```python
from build123d import *

# Parameters (mm, degrees)
SKETCH1_W                        = 69.85
SKETCH1_H                        = 19.05
MAIN_BODY_DEPTH                  = 3.175
CHIN_FEATURE_DEPTH               = 3.175
SKETCH10_W                       = 3.2258
SKETCH10_H                       = 6.35
CUT_FOR_TABS_DEPTH               = 4.175
CUT_FOR_LIP_MOTOR_APERTURE_DEPTH = 4.175
SKETCH12_R                       = 0.381
CUT_EXTRUDE1_DEPTH               = 4.175


with BuildPart() as part:
    # Sketch1 → main body (new body)
    with BuildSketch(Plane.XY):
        Rectangle(SKETCH1_W, SKETCH1_H)
    extrude(amount=MAIN_BODY_DEPTH)

    # Sketch9 → chin feature (add)
    with BuildSketch(Plane.XY.offset(3.175)):
        Polygon((-34.925, -9.525), (-34.925, -12.065), (-21.214947133, -17.145), (0, -17.145), (0, -9.525), align=None)
    chin_feature = extrude(amount=-CHIN_FEATURE_DEPTH)

    # mirror of chin feature: chin feature across plane
    add(chin_feature.mirror(Plane(origin=(0, 0, 0), x_dir=(0, 0, 1), z_dir=(1, 0, 0))))

    # Sketch10 → cut for tabs (cut, through all)
    with BuildSketch(Plane.XY.offset(3.175)):
        with Locations((-30.076100278, -4.050352196)):
            Rectangle(SKETCH10_W, SKETCH10_H)
        with Locations((19.20572281, -4.050352196)):
            Rectangle(SKETCH10_W, SKETCH10_H)
    extrude(amount=-CUT_FOR_TABS_DEPTH, mode=Mode.SUBTRACT)

    # Sketch11 → cut for lip motor aperture (cut, through all)
    with BuildSketch(Plane.XY.offset(3.175)):
        with BuildLine():
            Line((-23.576637278, 18.516146957), (-26.370637278, 18.516146957))
            Line((-26.370637278, 18.516146957), (-26.370637278, 14.520081328))
            ThreePointArc((-26.370637278, 14.520081328), (-23.470211189, 1.422172556), (-20.782637278, 14.565407781))
            Line((-20.782637278, 14.565407781), (-20.782637278, 18.516146957))
            Line((-20.782637278, 18.516146957), (-23.576637278, 18.516146957))
        make_face()
        with BuildLine():
            Line((23.530508447, 18.585729376), (20.736508447, 18.585729376))
            Line((20.736508447, 18.585729376), (20.736508447, 14.589663746))
            ThreePointArc((20.736508447, 14.589663746), (23.636934536, 1.491754974), (26.324508447, 14.634990199))
            Line((26.324508447, 14.634990199), (26.324508447, 18.585729376))
            Line((26.324508447, 18.585729376), (23.530508447, 18.585729376))
        make_face()
    extrude(amount=-CUT_FOR_LIP_MOTOR_APERTURE_DEPTH, mode=Mode.SUBTRACT)

    # Sketch12 → Cut-Extrude1 (cut, through all)
    with BuildSketch(Plane.XY.offset(3.175)):
        with Locations((0.018631462, 8.255)):
            Circle(SKETCH12_R)
    extrude(amount=-CUT_EXTRUDE1_DEPTH, mode=Mode.SUBTRACT)


solid = part.part
```
Here's how the part is built. I have some questions about the finished solid (model axes, mm). A direction names the side the tool comes from. Coordinates: 2 decimals unless noted, no trailing zeros. Order: outer loops, then holes, each group sorted by start corner. A loop starts at its lowest first (then second) coordinate and runs counter-clockwise, first axis right, second up. Notation, with made-up numbers: M -13.75,20 L -2.75,20 A30 cw -2.75,42 Z; hole C -14,52.5 d9. An arc over 180 degrees is marked long. Answer as a JSON object with one key per item and string values. Group by question number.
(1) If we mould it in two halves opening along X, with no side actions, what happens to faces 3 (the face through (17.593, -4, 2)), 4 (the face through (-33, 9.525, 2)), 5 (the face through (34.925, -1, 2))? For each: released by +X, released by -X, zero draft, split by the parting line, or undercut.
(2) Suppose I cut it at C-C, the plane y = 2.25. Please give me the cut outline in (x, z) (3 decimals).
(3) Suppose I cut it at A-A, the plane y = -3.75. Please give me the cut outline in (x, z) (3 decimals).
(4) I need wall thicknesses on probe 1 along X at (y, z) = (-5.5, 0.75) (3 decimals); probe 2 along X at (y, z) = (8.5, 0.65) (3 decimals); probe 3 along X at (y, z) = (7.25, 1.7) (3 decimals). Which ranges of each line are inside material? Lowest first, please.
(5) Which directions (+Z, -Z, +X, -X, +Y, -Y) give clear straight access to the entire face, cutting with the end or side of a thin tool? Please do faces 1 (the face through (-34.925, -1, 2)), 2 (the face through (-28.463, -4, 2)).
(6) For pin 1 (1.6 mm diameter, centred on x = 19, z = 2.5, fed in from +Y), with a flat end and sliding along its axis, tell me the tip position at first contact or that it passes through.
(7) Suppose I cut it at B-B, the plane z = 1.5. Please give me the cut outline in (x, y) (3 decimals), then the cut area to 3 significant figures.
(8) Suppose I cut it at D-D, the plane y = -13.25. Please give me the cut outline in (x, z) (3 decimals), then the cut area to 3 significant figures.
Values found:
{
 "1": {"face 3": "undercut", "face 4": "zero draft", "face 5": "released by +X"},
 "2": {"outline": "M -34.925,0 L -26.793,0 L -26.793,3.175 L -34.925,3.175 Z; M -20.259,0 L 20.446,0 L 20.446,3.175 L -20.259,3.175 Z; M 26.716,0 L 34.925,0 L 34.925,3.175 L 26.716,3.175 Z"},
 "3": {"outline": "M -34.925,0 L -31.689,0 L -31.689,3.175 L -34.925,3.175 Z; M -28.463,0 L 17.593,0 L 17.593,3.175 L -28.463,3.175 Z; M 20.819,0 L 34.925,0 L 34.925,3.175 L 20.819,3.175 Z"},
 "4": {"probe 1": "x = -34.925 to -31.689, -28.463 to 17.593, 20.819 to 34.925", "probe 2": "x = -34.925 to -30.38, -16.671 to -0.273, 0.31 to 16.725, 30.438 to 34.925", "probe 3": "x = -34.925 to -30.306, -16.746 to 16.812, 30.351 to 34.925"},
 "5": {"face 1": "+Z, -Z, -X, +Y, -Y", "face 2": "+Z, -Z"},
 "6": {"pin 1": "stops at y = 4.1"},
 "7": {"outline": "M -34.925,-12.065 L -21.215,-17.145 L 21.215,-17.145 L 34.925,-12.065 L 34.925,9.525 L 30.338,9.525 A6.858 cw long 16.825,9.525 L -16.782,9.525 A6.858 cw long -30.27,9.525 L -34.925,9.525 Z; hole M -31.689,-7.225 L -28.463,-7.225 L -28.463,-0.875 L -31.689,-0.875 Z; hole C 0.019,8.255 d0.762; hole M 17.593,-7.225 L 20.819,-7.225 L 20.819,-0.875 L 17.593,-0.875 Z", "area": "1,570 mm^2"},
 "8": {"outline": "M -31.727,0 L 31.727,0 L 31.727,3.175 L -31.727,3.175 Z", "area": "201 mm^2"}
}
